from build123d import *

# Parameters (mm, degrees)
SKETCH_1_W                   = 3
SKETCH_1_H                   = 1
SKETCH_1_H_2                 = 2
SKETCH_1_W_2                 = 30
EXTRUDE_1_DEPTH              = 1
SKETCH_2_W                   = 20
SKETCH_2_H                   = 12
SKETCH_2_W_2                 = 18
SKETCH_2_H_2                 = 10
EXTRUDE_4_DEPTH              = 4
SKETCH_8_W                   = 18
SKETCH_8_H                   = 4
CUT_EXTRUDE_2_DEPTH          = 4
SKETCH_9_W                   = 1.25
SKETCH_9_H                   = 1
EXTRUDE_5_DEPTH              = 2
EXTRUDE_6_DEPTH              = 1
HOLE_WIZARD_M2_1_D           = 1.6
HOLE_WIZARD_M2_1_DEPTH       = 5.5
HOLE_WIZARD_M2_1_CSINK_D     = 2.05
HOLE_WIZARD_M2_1_CSINK_ANGLE = 90
HOLE_WIZARD_M2_1_TIP         = 0.480688495
HOLE_WIZARD_M2_2_D           = 1.6
HOLE_WIZARD_M2_2_CSINK_D     = 2.05
HOLE_WIZARD_M2_2_CSINK_ANGLE = 90
CHAMFER_1_SIZE               = 0.2
CHAMFER_2_SIZE               = 0.2
CHAMFER_3_SIZE               = 0.2
CHAMFER_4_SIZE               = 0.2
CHAMFER_5_SIZE               = 0.2
SKETCH_16_R                  = 0.8
EXTRUDE_7_DEPTH              = 3
SKETCH_17_R                  = 0.8
CUT_EXTRUDE_3_DEPTH          = 22


with BuildPart() as part:
    # 草图1 → 凸台-拉伸1 (new body)
    with BuildSketch(Plane(origin=(0, 0, 0), x_dir=(1, 0, 0), z_dir=(0, 1, 0))):
        with BuildLine():
            ThreePointArc((-15, 4), (-16.5, 5.5), (-18, 4))
            Line((-18, 4), (-15, 4))
        make_face()
        with BuildLine():
            ThreePointArc((-15, 4), (-16.5, 2.5), (-18, 4))
            Line((-18, 4), (-18, -1))
            Line((-18, -1), (-15, -1))
            Line((-15, -1), (-15, -2))
            Line((-15, -2), (15, -2))
            Line((15, -2), (15, -1))
            Line((15, -1), (18, -1))
            Line((18, -1), (18, 4))
            ThreePointArc((18, 4), (16.5, 2.5), (15, 4))
            Line((15, 4), (-15, 4))
        make_face()
        with BuildLine():
            Line((-15, 4), (-18, 4))
            ThreePointArc((-18, 4), (-16.5, 2.5), (-15, 4))
        make_face()
        with Locations((-16.5, -1.5)):
            Rectangle(SKETCH_1_W, SKETCH_1_H)
        with BuildLine():
            ThreePointArc((18, 4), (16.5, 5.5), (15, 4))
            Line((15, 4), (18, 4))
        make_face()
        with BuildLine():
            Line((18, 4), (15, 4))
            ThreePointArc((15, 4), (16.5, 2.5), (18, 4))
        make_face()
        with Locations((-16.5, -3)):
            Rectangle(SKETCH_1_W, SKETCH_1_H_2)
        Polygon((-18, -4), (-18, -2), (-19, -2), (-19, -8), (19, -8), (19, -2), (18, -2), (18, -4), (15, -4), (-15, -4), align=None)
        with Locations((0, -3)):
            Rectangle(SKETCH_1_W_2, SKETCH_1_H_2)
        with Locations((16.5, -1.5)):
            Rectangle(SKETCH_1_W, SKETCH_1_H)
        with Locations((16.5, -3)):
            Rectangle(SKETCH_1_W, SKETCH_1_H_2)
    extrude(amount=EXTRUDE_1_DEPTH)

    # 草图2 → 凸台-拉伸4 (add)
    with BuildSketch(Plane(origin=(0, 1, 0), x_dir=(1, 0, 0), z_dir=(0, 1, 0))):
        with Locations((0, -2)):
            Rectangle(SKETCH_2_W, SKETCH_2_H)
        with Locations((0, -2)):
            Rectangle(SKETCH_2_W_2, SKETCH_2_H_2, mode=Mode.SUBTRACT)
    extrude(amount=EXTRUDE_4_DEPTH)

    # 草图8 → 切除-拉伸2 (cut)
    with BuildSketch(Plane.XY.offset(8)):
        with Locations((0, 3)):
            Rectangle(SKETCH_8_W, SKETCH_8_H)
    extrude(amount=-CUT_EXTRUDE_2_DEPTH, mode=Mode.SUBTRACT)

    # 草图9 → 凸台-拉伸5 (add)
    with BuildSketch(Plane.XY.offset(8)):
        with Locations((-8.375, 1.5)):
            Rectangle(SKETCH_9_W, SKETCH_9_H)
        with Locations((8.375, 1.5)):
            Rectangle(SKETCH_9_W, SKETCH_9_H)
    extrude(amount=-EXTRUDE_5_DEPTH)

    # 草图10 → 凸台-拉伸6 (add)
    with BuildSketch(Plane.XZ):
        Polygon((-13, 8), (-19, 8), (-19, 2), (-18, 2), (-13, 2), (-13, 5), (-13, 6.5), align=None)
        with BuildLine():
            ThreePointArc((-11.5, 5), (-12.560660172, 5.439339828), (-13, 6.5))
            Line((-13, 6.5), (-13, 5))
            Line((-13, 5), (-11.5, 5))
        make_face()
        with BuildLine():
            ThreePointArc((-11.5, 8), (-12.560660172, 7.560660172), (-13, 6.5))
            ThreePointArc((-13, 6.5), (-12.560660172, 5.439339828), (-11.5, 5))
            Line((-11.5, 5), (-11.5, 8))
        make_face()
        with BuildLine():
            ThreePointArc((-10, 6.5), (-10.439339828, 7.560660172), (-11.5, 8))
            Line((-11.5, 8), (-11.5, 5))
            ThreePointArc((-11.5, 5), (-10.439339828, 5.439339828), (-10, 6.5))
        make_face()
        with BuildLine():
            Line((-11.5, 8), (-13, 8))
            Line((-13, 8), (-13, 6.5))
            ThreePointArc((-13, 6.5), (-12.560660172, 7.560660172), (-11.5, 8))
        make_face()
        with BuildLine():
            ThreePointArc((13, 6.5), (12.560660172, 7.560660172), (11.5, 8))
            Line((11.5, 8), (11.5, 5))
            ThreePointArc((11.5, 5), (12.560660172, 5.439339828), (13, 6.5))
        make_face()
        with BuildLine():
            Line((11.5, 5), (11.5, 8))
            ThreePointArc((11.5, 8), (10, 6.5), (11.5, 5))
        make_face()
        with BuildLine():
            Line((13, 8), (11.5, 8))
            ThreePointArc((11.5, 8), (12.560660172, 7.560660172), (13, 6.5))
            Line((13, 6.5), (13, 8))
        make_face()
        with BuildLine():
            ThreePointArc((13, 6.5), (12.560660172, 5.439339828), (11.5, 5))
            Line((11.5, 5), (13, 5))
            Line((13, 5), (13, 6.5))
        make_face()
        Polygon((19, 8), (13, 8), (13, 6.5), (13, 5), (13, 2), (18, 2), (19, 2), align=None)
    extrude(amount=EXTRUDE_6_DEPTH)

    # M2 螺纹孔1
    with Locations(Plane(origin=(0, 1, 0), x_dir=(1, 0, 0), z_dir=(0, 1, 0))):
        with Locations((-16.5, 4), (16.5, 4)):
            CounterSinkHole(HOLE_WIZARD_M2_1_D / 2, HOLE_WIZARD_M2_1_CSINK_D / 2, depth=HOLE_WIZARD_M2_1_DEPTH, counter_sink_angle=HOLE_WIZARD_M2_1_CSINK_ANGLE)
            with Locations((0, 0, -(HOLE_WIZARD_M2_1_DEPTH + HOLE_WIZARD_M2_1_TIP / 2))):  # 118° drill point
                Cone(0, HOLE_WIZARD_M2_1_D / 2, HOLE_WIZARD_M2_1_TIP, mode=Mode.SUBTRACT)

    # M2 螺纹孔2 (through all)
    with Locations(Plane(origin=(0, -1, 0), x_dir=(-1, 0, 0), z_dir=(0, -1, 0))):
        with Locations((11.5, -6.5), (-11.5, -6.5)):
            CounterSinkHole(HOLE_WIZARD_M2_2_D / 2, HOLE_WIZARD_M2_2_CSINK_D / 2, counter_sink_angle=HOLE_WIZARD_M2_2_CSINK_ANGLE)

    # 倒角1
    chamfer_1_edges = [part.edges().sort_by_distance(p)[0] for p in [
        (-10, 5, 2),
        (-9.5, 5, 8),
        (10, 5, 2),
        (0, 5, -4),
        (0, 5, -3),
        (-9, 5, 2.5),
        (9, 5, 2.5),
        (9.5, 5, 8),
    ]]
    chamfer(chamfer_1_edges, length=CHAMFER_1_SIZE)

    # 倒角2
    chamfer_2_edges = [part.edges().sort_by_distance(p)[0] for p in [
        (-18, 1, -1),
        (-18.5, 1, 2),
        (-19, 1, 5),
        (-14.5, 1, 8),
        (19, 1, 5),
        (18.5, 1, 2),
        (12.5, 1, -4),
        (14.5, 1, 8),
        (18, 1, -1),
        (-12.5, 1, -4),
        (16.5, 1, -5.5),
        (-16.5, 1, -5.5),
    ]]
    chamfer(chamfer_2_edges, length=CHAMFER_2_SIZE)

    # 倒角3
    chamfer_3_edges = [part.edges().sort_by_distance(p)[0] for p in [
        (7.75, 1.5, 8),
        (-9, 3.4, 8),
        (-10, 2.8, 8),
        (10, 2.8, 8),
        (0, 1, 8),
        (-7.75, 1.5, 8),
        (-8.375, 2, 8),
        (9, 3.4, 8),
        (8.375, 2, 8),
    ]]
    chamfer(chamfer_3_edges, length=CHAMFER_3_SIZE)

    # 倒角4
    chamfer_4_edges = [part.edges().sort_by_distance(p)[0] for p in [
        (-19, -0.1, 8),
        (19, -0.1, 8),
        (-19, -0.1, 2),
        (19, -0.1, 2),
    ]]
    chamfer(chamfer_4_edges, length=CHAMFER_4_SIZE)

    # 倒角5
    chamfer_5_edges = [part.edges().sort_by_distance(p)[0] for p in [
        (-10, 2.8, -4),
        (10, 2.8, -4),
    ]]
    chamfer(chamfer_5_edges, length=CHAMFER_5_SIZE)

    # 草图16 → 凸台-拉伸7 (add)
    with BuildSketch(Plane(origin=(0, 1, 0), x_dir=(1, 0, 0), z_dir=(0, 1, 0))):
        with Locations(Location((16.5, 4, 0), (0, 0, 270))):
            Circle(SKETCH_16_R)
        with Locations(Location((11.5, -6.5, 0), (0, 0, 270))):
            Circle(SKETCH_16_R)
        with Locations(Location((-11.5, -6.5, 0), (0, 0, 270))):
            Circle(SKETCH_16_R)
        with Locations(Location((-16.5, 4, 0), (0, 0, 270))):
            Circle(SKETCH_16_R)
    extrude(amount=-EXTRUDE_7_DEPTH)

    # 草图17 → 切除-拉伸3 (cut, through all)
    with BuildSketch(Plane(origin=(0, 1, 0), x_dir=(1, 0, 0), z_dir=(0, 1, 0))):
        with Locations(Location((-16.5, 4, 0), (0, 0, 270))):
            Circle(SKETCH_17_R)
        with Locations(Location((-11.5, -6.5, 0), (0, 0, 270))):
            Circle(SKETCH_17_R)
        with Locations(Location((11.5, -6.5, 0), (0, 0, 270))):
            Circle(SKETCH_17_R)
        with Locations(Location((16.5, 4, 0), (0, 0, 270))):
            Circle(SKETCH_17_R)
    extrude(amount=-CUT_EXTRUDE_3_DEPTH, mode=Mode.SUBTRACT)


solid = part.part
Read the model definition and answer for the solid it produces. Units are mm, in the model's axes. A direction names the side the tool comes from. Round coordinates to 2 decimals unless told otherwise and drop trailing zeros. Loops run counter-clockwise (first coordinate to the right, second up) from the corner with the lowest first, then second, coordinate; pieces in that order, holes last.
Q1. Section A-A on x = 8.5 is taken. Write down the section's boundary in (y, z), and give its area (3 significant figures).
Q2. Each of these flat-tipped pins is pushed along its axis until it touches: pin 1 (7 mm diameter, centred on x = 5, z = 1.5, fed in from -Y); pin 2 (0.5 mm diameter, centred on x = 8, y = 1.5, fed in from -Z); pin 3 (7 mm diameter, centred on x = -14, z = 4, fed in from +Y); pin 4 (2 mm diameter, centred on x = 9, y = 2.5, fed in from +Z). Where does it stop, or does it pass through?
Q3. Consider probe 1 along X at (y, z) = (0.65, 6.5); probe 2 along Z at (x, y) = (-11.5, -0.3); probe 3 along X at (y, z) = (2.75, -2.25). Determine where each line is inside the solid, lowest interval first.
Q4. Section B-B on z = -1.5 is taken. Write down the section's boundary in (x, y), and give its area (3 significant figures).
Q5. Determine the mould class of faces 6 (the face through (-14, 1, 1)), 7 (the face through (0, 3, -3)), 8 (the face through (-10, 3, 2)) for opening direction X: released by +X, released by -X, zero draft, split by the parting line, or undercut.
Q6. Section C-C on y = 4.25 is taken. Write down the section's boundary in (x, z).
Q7. Section D-D on x = -16.5 is taken. Write down the section's boundary in (y, z) (3 decimals), and give its area (3 significant figures).
Q8. Which of the six approach directions +Z, -Z, +X, -X, +Y, -Y give full straight-line access (tool end or side, diameter ignored) to faces 1 (the face through (-10.96, 0.12, 5.91)), 2 (the face through (-12.3, -0.5, 5)), 3 (the face through (-8.4, 1.5, 6)), 4 (the face through (-16, -1, 5)), 5 (the face through (-7.75, 1.5, 6.9))?
Output:
1. outline: (0, -4) - (4.8, -4) - (5, -3.8) - (5, -3.2) - (4.8, -3) - (1, -3) - (1, 6) - (2, 6) - (2, 7.8) - (1.8, 8) - (0, 8) - close
1. area: 17.9 mm2
2. pin 1: stops at y = 0
2. pin 2: stops at z = -4
2. pin 3: stops at y = 1
2. pin 4: stops at z = 8
3. probe 1: x = -19 to -12.3, -10.7 to 10.7, 12.3 to 19
3. probe 2: z = 5 to 5.7, 7.3 to 8
3. probe 3: x = -10 to -9, 9 to 10
4. outline: (-18, 0) - (18, 0) - (18, 0.8) - (17.8, 1) - (10, 1) - (10, 4.8) - (9.8, 5) - (9.2, 5) - (9, 4.8) - (9, 1) - (-9, 1) - (-9, 4.8) - (-9.2, 5) - (-9.8, 5) - (-10, 4.8) - (-10, 1) - (-17.8, 1) - (-18, 0.8) - close
4. area: 43.9 mm2
5. face 6: zero draft
5. face 7: undercut
5. face 8: released by -X
6. outline: (-10, -3.8) - (-9.8, -4) - (9.8, -4) - (10, -3.8) - (10, 7.8) - (9.8, 8) - (9.2, 8) - (9, 7.8) - (9, -3) - (-9, -3) - (-9, 7.8) - (-9.2, 8) - (-9.8, 8) - (-10, 7.8) - close
7. outline: (-1, 2) - (0, 2) - (0, -3.2) - (0.775, -3.2) - (1, -2.975) - (1, 7.8) - (0.8, 8) - (-1, 8) - close; (0, -5.5) - (0.8, -5.5) - (1, -5.3) - (1, -5.025) - (0.775, -4.8) - (0, -4.8) - close
7. area: 17.8 mm2
8. face 1: +Y, -Y
8. face 2: -Z, -Y
8. face 3: +Y
8. face 4: +Z, -Z, +X, -X, -Y
8. face 5: +Z, +Y
